from build123d import *
from build123d.topology import SkipClean

# Parameters (mm, degrees)
SKETCH_1_R          = 47.5
SKETCH_1_R_2        = 2
EXTRUDE_1_DEPTH     = 14
EXTRUDE_START       = 5.2
SKETCH_2_R          = 9
SKETCH_2_R_2        = 2
EXTRUDE_2_DEPTH     = 5.2
SKETCH_4_R          = 40
SKETCH_4_R_2        = 9
CUT_EXTRUDE_3_DEPTH = 3
CUT_EXTRUDE_START   = -3
SKETCH_3_R          = 40
CUT_EXTRUDE_4_DEPTH = 3


with BuildPart() as part:
    # 草图1 → 凸台-拉伸1 (new body)
    with BuildSketch(Plane(origin=(0, 0, 0), x_dir=(1, 0, 0), z_dir=(0, 1, 0))):
        with Locations(Location((0, 0, 0), (0, 0, 270))):
            Circle(SKETCH_1_R)
        with Locations(Location((0, 0, 0), (0, 0, 270))):
            Circle(SKETCH_1_R_2, mode=Mode.SUBTRACT)
    extrude(amount=EXTRUDE_1_DEPTH)

    # 草图2 → 凸台-拉伸2 (add)
    with SkipClean():  # the faces are left unmerged after this step: merging them gives an invalid solid
        with BuildSketch(Plane(origin=(0, 0, 0), x_dir=(-1, 0, 0), z_dir=(0, -1, 0)).offset(EXTRUDE_START)):
            with Locations(Location((0, 0, 0), (0, 0, 270))):
                Circle(SKETCH_2_R)
            with Locations(Location((0, 0, 0), (0, 0, 90))):
                Circle(SKETCH_2_R_2, mode=Mode.SUBTRACT)
        extrude(amount=-EXTRUDE_2_DEPTH)

    # 草图4 → 切除-拉伸3 (cut)
    with SkipClean():  # the faces are left unmerged after this step: merging them gives an invalid solid
        with BuildSketch(Plane.XZ):
            with Locations(Location((0, 0, 0), (0, 0, 270))):
                Circle(SKETCH_4_R)
            with Locations(Location((0, 0, 0), (0, 0, 270))):
                Circle(SKETCH_4_R_2, mode=Mode.SUBTRACT)
        extrude(amount=-CUT_EXTRUDE_3_DEPTH, mode=Mode.SUBTRACT)

    # 草图3 → 切除-拉伸4 (cut)
    with BuildSketch(Plane(origin=(0, 14, 0), x_dir=(1, 0, 0), z_dir=(0, 1, 0)).offset(CUT_EXTRUDE_START)):
        with Locations(Location((0, 0, 0), (0, 0, 90))):
            Circle(SKETCH_3_R)
    extrude(amount=CUT_EXTRUDE_4_DEPTH, mode=Mode.SUBTRACT)


solid = part.part
Build history of the part. All positions in model axes, mm. A direction names the side the tool comes from. Coordinates: 2 decimals unless noted, no trailing zeros. Write each loop counter-clockwise with the first axis right and the second up, starting at its lowest first coordinate (ties: lowest second). Pieces come first, ordered by that corner, then holes. Notation, with made-up numbers: (-15.75, 23.25) -> (42.25, 23.25) arc R30 cw to (42.25, 60.25) -> close; hole circle Ø10 at (-6, -12). An arc over 180 degrees is marked (long way). Use CSV: the item, a comma, the result in double quotes. Start each with the question number.
Q1. Flat gauge pins, fed straight in: pin 1 Ø3 at (x, y) = (24.5, 8.5) entering from +Z; pin 2 Ø10 at (x, y) = (10, 8) entering from -Z; pin 3 Ø1 at (y, z) = (4.5, -12) entering from +X. Where does each tip first touch, or does it go through?
Q2. Cut at D-D, the plane x = 32. List the corners of the cut face in (y, z).
Q3. Drill centre lines: probe 1 along X at (y, z) = (1.55, 0); probe 2 along X at (y, z) = (12.8, 0); probe 3 along X at (y, z) = (4, 0). Where is each one in solid material? Low to high.
Q4. 3-axis set-ups, long thin cutter, end or side, ignore diameter. For faces 5 (the cylindrical face through (39.05, 12.48, 8.67)), 6 (the flat face through (9.4, 3, 0.6)), 7 (the flat face through (-35, 14, -21)): which of +Z, -Z, +X, -X, +Y, -Y reach the whole face in a straight line?
Q5. Pull direction X, two halves, no side cores. Call faces 1 (the flat face through (-1, 11, -8)), 2 (the cylindrical face through (-46.37, 6.9, -10.3)), 3 (the flat face through (2, -5.2, 2)), 4 (the cylindrical face through (-8.98, -1.16, 0.59)): released by +X, released by -X, zero draft, split by the parting line, or undercut.
Checked values:
1,pin 1,"stops at z = 41.56"
1,pin 2,"stops at z = -47.24"
1,pin 3,"stops at x = 46.09"
2,outline,"(0, -35.1) -> (14, -35.1) -> (14, -24) -> (11, -24) -> (11, 24) -> (14, 24) -> (14, 35.1) -> (0, 35.1) -> (0, 24) -> (3, 24) -> (3, -24) -> (0, -24) -> close"
3,probe 1,"x = -47.5 to -40, -9 to -2, 2 to 9, 40 to 47.5"
3,probe 2,"x = -47.5 to -40, 40 to 47.5"
3,probe 3,"x = -47.5 to -2, 2 to 47.5"
4,face 5,"+Y"
4,face 6,"-Y"
4,face 7,"+Z, -Z, +X, -X, +Y"
5,face 1,"undercut"
5,face 2,"split by the parting line"
5,face 3,"zero draft"
5,face 4,"undercut"
